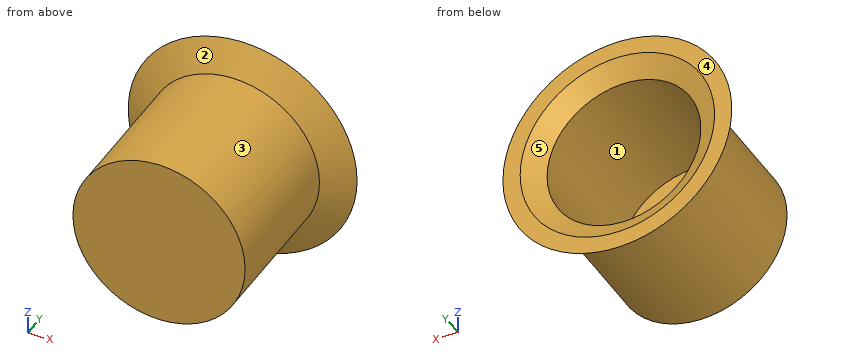
from build123d import *

# Parameters (mm, degrees)
F2_T = -2.54


with BuildPart() as f1:
    # F0 (on Top) → F1 (revolve)
    with BuildSketch(Plane.XY):
        Polygon((31.655497849, 44.5790737867), (0, 44.5790737867), (0, 0), (23.8142292947, 0), (23.8142292947, 39.6419800818), align=None)
    revolve(axis=Axis((0, 22.2895368934, 0), (0, -1, 0)))

    # F2
    f2_openings = [f1.faces().sort_by_distance(p)[0] for p in [
        (0, 44.579074, 0),
    ]]
    offset(amount=F2_T, openings=f2_openings, kind=Kind.INTERSECTION)


solid = f1.part
Work out the finished part from the listing and answer in its coordinate system (mm). Face numbers are marked on the shaded views. A direction names the side the tool comes from. Give positions to 0.01 mm unless a question says otherwise; leave off trailing zeros. Order: outer loops, then holes, each group sorted by start corner. A loop starts at its lowest first (then second) coordinate and runs counter-clockwise, first axis right, second up. Notation, with made-up numbers: M 6.5,25.25 L 33.5,25.25 A10 ccw 33.5,41.25 Z; hole C 75.25,-8.75 d5. An arc over 180 degrees is marked long. Return JSON: item names as keys, results as strings.
Q1. Find section B-B, the plane x = 0. Write down the section's boundary in (y, z).
Answer below:
{"outline": "M 0,-23.81 L 39.64,-23.81 L 44.58,-31.66 L 44.58,-26.89 L 41.04,-21.27 L 2.54,-21.27 L 2.54,21.27 L 41.04,21.27 L 44.58,26.89 L 44.58,31.66 L 39.64,23.81 L 0,23.81 Z"}
Q2. Each of these flat-tipped pins is pushed along its axis until it touches: pin 1 (5 mm diameter, centred on x = -16.5, z = 10.5, fed in from +Y); pin 2 (6 mm diameter, centred on x = -14.5, y = 31.5, fed in from -Z); pin 3 (6 mm diameter, centred on x = 6.5, y = 14.5, fed in from +Z). Where does it stop, or does it pass through?
Answer below:
{"pin 1": "stops at y = 41.54", "pin 2": "stops at z = -20.85", "pin 3": "stops at z = 23.56"}
Q3. Find section C-C, the plane y = 11.5. Write down the section's boundary in (x, z), and give its area (3 significant figures).
Answer below:
{"outline": "C 0,0 d47.63; hole C 0,0 d42.55", "area": "360 mm^2"}
Q4. Which of the six approach directions +Z, -Z, +X, -X, +Y, -Y give full straight-line access (tool end or side, diameter ignored) to the marked faces 1 and 2?
Answer below:
{"face 1": "+Y", "face 2": "-Y"}
Q5. The mould has two halves that part along X. Classify the marked faces 3, 4 and 5: pulls with the +X half, pulls with the -X half, needs draft (parallel to the pull), parting line crosses it, or undercut.
Answer below:
{"face 3": "parting line crosses it", "face 4": "needs draft", "face 5": "undercut"}
Q6. Find the intervals of material crossed by line 1 along Z through (x, y) = (0, 11); line 2 along X through (y, z) = (13.5, 6); line 3 along X through (y, z) = (28, 16.5), in increasing order. Write a range as [from, to].
Answer below:
{"line 1": "z = [-23.81, -21.27], [21.27, 23.81]", "line 2": "x = [-23.05, -20.41], [20.41, 23.05]", "line 3": "x = [-17.17, -13.43], [13.43, 17.17]"}
Q7. Find section A-A, the plane z = 0. Write down the section's boundary in (x, y).
Answer below:
{"outline": "M -31.66,44.58 L -23.81,39.64 L -23.81,0 L 23.81,0 L 23.81,39.64 L 31.66,44.58 L 26.89,44.58 L 21.27,41.04 L 21.27,2.54 L -21.27,2.54 L -21.27,41.04 L -26.89,44.58 Z"}
